```python
from build123d import *

# Parameters (mm, degrees)
F1_DEPTH = 95.25
F2_R     = 1.5875
F3_DEPTH = 3.175
F4_DEPTH = 3.175
F5_R     = 5.08
F6_R     = 2.38125
F7_DEPTH = 3.175
F9_DEPTH = 12.7


with BuildPart() as f1:
    # F0 (on Top) → F1 (new body)
    with BuildSketch(Plane.XY):
        with BuildLine():
            Line((-92.1331368885, -117.6278676055), (-93.9624351915, -120.2229191885))
            Line((-93.9624351915, -120.2229191885), (-83.2106191336, -127.802066747))
            ThreePointArc((-83.2106191336, -127.802066747), (-76.6288041341, -128.2490988663), (-73.2020225275, -122.611963581))
            Line((-73.2020225275, -122.611963581), (-73.2020225275, -95.6804940123))
            ThreePointArc((-73.2020225275, -95.6804940123), (-72.9539595945, -93.922977574), (-72.2291519666, -92.3027759964))
            Line((-72.2291519666, -92.3027759964), (-10.2165459343, 6.4176642302))
            ThreePointArc((-10.2165459343, 6.4176642302), (6.4176642302, 10.2165459343), (10.2165459343, -6.4176642302))
            Line((10.2165459343, -6.4176642302), (3.7988817041, -16.6342101646))
            Line((3.7988817041, -16.6342101646), (6.4874464236, -18.3230691725))
            Line((6.4874464236, -18.3230691725), (12.9051106539, -8.1065232382))
            ThreePointArc((12.9051106539, -8.1065232382), (8.1065232382, 12.9051106539), (-12.9051106539, 8.1065232382))
            Line((-12.9051106539, 8.1065232382), (-74.9177166862, -90.6139169884))
            ThreePointArc((-74.9177166862, -90.6139169884), (-76.004928128, -93.0442193549), (-76.3770225275, -95.6804940123))
            Line((-76.3770225275, -95.6804940123), (-76.3770225275, -122.611963581))
            ThreePointArc((-76.3770225275, -122.611963581), (-78.0904133308, -125.4305312236), (-81.3813208306, -125.207015164))
            Line((-81.3813208306, -125.207015164), (-92.1331368885, -117.6278676055))
        make_face()
    extrude(amount=F1_DEPTH)

    # F2 (on face) → F3 (cut, through all)
    with BuildSketch(Plane(origin=(-87.8063185468, -124.562475984, 0), x_dir=(0.8173390813, -0.5761569458, 0), z_dir=(-0.5761569458, -0.8173390813, 0))):
        with Locations((0, 85.725)):
            Circle(F2_R)
        with Locations((0, 9.525)):
            Circle(F2_R)
    extrude(amount=-F3_DEPTH, mode=Mode.SUBTRACT)

    # F2 (on face) → F4 (cut, through all)
    with BuildSketch(Plane(origin=(-87.8063185468, -124.562475984, 0), x_dir=(0.8173390813, -0.5761569458, 0), z_dir=(-0.5761569458, -0.8173390813, 0))):
        Polygon((5.6227574559, 69.85), (-7.5319005121, 75.2988377387), (-7.5319005121, 19.9511622613), (5.6227574559, 25.4), align=None)
    extrude(amount=-F4_DEPTH, mode=Mode.SUBTRACT)

    # F5
    f5_edges = [f1.edges().sort_by_distance(p)[0] for p in [
        (-93.047786, -118.925393, 95.25),
        (-93.047786, -118.925393, 75.298838),
        (-82.29597, -126.504541, 69.85),
        (-82.29597, -126.504541, 25.4),
        (-93.047786, -118.925393, 19.951162),
        (-93.047786, -118.925393, 0),
    ]]
    fillet(f5_edges, radius=F5_R)

    # F6 (on face) → F7 (cut, through all)
    with BuildSketch(Plane(origin=(12.9051106539, -8.1065232382, 0), x_dir=(0.531924097, 0.8467920377, 0), z_dir=(0.8467920377, -0.531924097, 0))):
        with Locations((-5.377555266, 79.375)):
            Circle(F6_R)
        with Locations((-5.377555266, 15.875)):
            Circle(F6_R)
    extrude(amount=-F7_DEPTH, mode=Mode.SUBTRACT)

    # F8 (on face) → F9 (cut)
    with BuildSketch(Plane(origin=(12.9051106539, -8.1065232382, 0), x_dir=(0.531924097, 0.8467920377, 0), z_dir=(0.8467920377, -0.531924097, 0))):
        with BuildLine():
            Line((-3.175, 66.2270688534), (-12.065, 66.2270688534))
            Line((-12.065, 66.2270688534), (-12.065, 29.0229311466))
            Line((-12.065, 29.0229311466), (-3.175, 29.0229311466))
            ThreePointArc((-3.175, 29.0229311466), (-0.9299359697, 29.9528671164), (0, 32.1979311466))
            Line((0, 32.1979311466), (0, 63.0520688534))
            ThreePointArc((0, 63.0520688534), (-0.9299359697, 65.2971328836), (-3.175, 66.2270688534))
        make_face()
    extrude(amount=-F9_DEPTH, mode=Mode.SUBTRACT)


solid = f1.part
```
Work out the finished part from the listing and answer in its coordinate system (mm). A direction names the side the tool comes from. Give positions to 0.01 mm unless a question says otherwise; leave off trailing zeros. Order: outer loops, then holes, each group sorted by start corner. A loop starts at its lowest first (then second) coordinate and runs counter-clockwise, first axis right, second up. Notation, with made-up numbers: M 72,23 L 88,23 A22 cw 88,61 Z; hole C 88.25,44.5 d11. An arc over 180 degrees is marked long. Return JSON: item names as keys, results as strings.
1) Each of these flat-tipped pins is pushed along its axis until it touches: pin 1 (13.5 mm diameter, centred on y = -111.5, z = 49.5, fed in from +X); pin 2 (5 mm diameter, centred on x = -54, z = 57.5, fed in from +Y); pin 3 (8 mm diameter, centred on y = -87, z = 49, fed in from -X). Where does it stop, or does it pass through?
Resolved:
{"pin 1": "x = -73.2", "pin 2": "y = -53.33", "pin 3": "x = -75.15"}
2) Section C-C, the plane x = 0 is taken. Write down the section's boundary in (y, z) (3 decimals).
Resolved:
{"outline": "M 12.065,0 L 15.24,0 L 15.24,95.25 L 12.065,95.25 Z"}
3) For a pull along X with two mould halves and no side action, classify faces 5 (the cylindrical face through (-78.05, -125.41, 46.96)), 6 (the cylindrical face through (-72.96, -93.95, 46.96)), 7 (the cylindrical face through (-82.964, -126.006, 69.243)) as +X half, -X half, draft (parallel to the pull), parting line (faces both ways), or undercut.
Resolved:
{"face 5": "undercut", "face 6": "+X half", "face 7": "-X half"}
4) Straight lines are drawn through the part: line 1 along X through (y, z) = (-122.5, 56); line 2 along X through (y, z) = (1.5, 51.5); line 3 along Y through (x, z) = (-66, 57). For each, find the intervals that lie inside material, in ascending order. Write a range as [from, to].
Resolved:
{"line 1": "[-76.38, -73.2]", "line 2": "[-17.06, -13.31], [11.97, 15.17]", "line 3": "[-82.39, -76.42]"}
5) A tool of negligible diameter and unlimited length cuts with its end or side. For faces 1 (the flat face through (-41.657, -43.634, 46.958)), 2 (the flat face through (-87.645, -122.761, 72.554)), 3 (the flat face through (-87.877, -120.628, 10.996)), 4 (the cylindrical face through (11.1, -8.04, 65.27)), from which of +Z, -Z, +X, -X, +Y, -Y can it reach the whole face along a straight path? Write none if from no direction.
Resolved:
{"face 1": "+Z, -Z, -Y", "face 2": "-X, +Y", "face 3": "+Z, -Z, +Y", "face 4": "-Y"}
6) Section D-D, the plane y = -62 is taken. Write down the section's boundary in (x, z), plus the area to 3 significant figures.
Resolved:
{"outline": "M -56.94,0 L -53.19,0 L -53.19,95.25 L -56.94,95.25 Z", "area": "357 mm^2"}
7) Section A-A, the plane y = 0 is taken. Write down the section's boundary in (x, z) (3 decimals).
Resolved:
{"outline": "M -17.997,0 L -14.248,0 L -14.248,95.25 L -17.997,95.25 Z; M 12.065,0 L 15.24,0 L 15.24,95.25 L 12.065,95.25 Z"}
